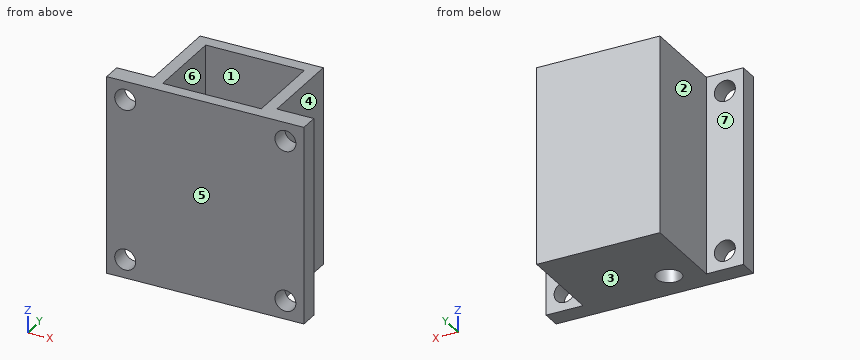
Autodesk Fusion 360 part; units mm, degrees
sketch "Esquisse1" plane through (0, 0, 0) normal (0, 0, 1) x (1, 0, 0)
  line L0 (8, 6.5) -> (-8, 6.5)
  line L1 (-8, 6.5) -> (-8, -6.5)
  line L2 (-8, -6.5) -> (8, -6.5)
  line L3 (8, -6.5) -> (8, 6.5)
  line L4 (8, 6.5) -> (-8, -6.5) construction
  line L5 (-8, 6.5) -> (8, -6.5) construction
  line L6 (-10, -8.5) -> (10, -8.5)
  line L7 (10, -8.5) -> (10, 8.5)
  line L8 (10, 8.5) -> (-10, 8.5)
  line L9 (-10, 8.5) -> (-10, -8.5)
  circle A0 centre (-5, -3.5) radius 2
  dimension "d1" = 16
  dimension "d2" = 13
  dimension "d3" = 2
  dimension "d15" = 4
  dimension "d16" = 3
  dimension "d18" = 3
extrude "Extrusion1" add sketch "Esquisse1" along normal blind 32 contours L6 L7 L8 L9
extrude "Extrusion2" add sketch "Esquisse1" along normal blind 3 contours L0 L1 L2 L3
sketch "Esquisse2" plane through (0, -8.5, 0) normal (0, -1, 0) x (1, 0, 0)
  line L0 (-10, 0) -> (10, 0)
  line L1 (10, 0) -> (10, 32)
  line L2 (10, 32) -> (-10, 32)
  line L3 (-10, 32) -> (-10, 0)
  line L4 (16, 32) -> (-16, 32)
  line L5 (-16, 32) -> (-16, 0)
  line L6 (-16, 0) -> (16, 0)
  line L7 (16, 0) -> (16, 32)
  line L8 (16, 32) -> (-16, 0) construction
  line L9 (-16, 32) -> (16, 0) construction
  line L10 (-10, 0) -> (10, 0)
  circle A0 centre (13, 29) radius 1.7
  line L11 (0, 16) -> (16, 16) construction
  line L12 (0, 16) -> (0, 32) construction
  circle A1 centre (13, 3) radius 1.7
  circle A2 centre (-13, 3) radius 1.7
  circle A3 centre (-13, 29) radius 1.7
  point P0 (0, 16)
  dimension "d8" = 6
  dimension "d9" = 6
  dimension "d10" = 3.4
  dimension "d11" = 3
  dimension "d12" = 3
extrude "Extrusion3" add sketch "Esquisse2" against normal blind 3 contours L3 L4 L5 L6 | L1 L4 L6 L7
equation "d9 = d8"
equation "d18 = d16"
Verification items for the finished model (mm, model axes). Face numbers are marked on the shaded views. A direction names the side the tool comes from. Coordinates: 2 decimals unless noted, no trailing zeros. Order: outer loops, then holes, each group sorted by start corner. A loop starts at its lowest first (then second) coordinate and runs counter-clockwise, first axis right, second up. Notation, with made-up numbers: M -13,48.25 L 21,48.25 A6 ccw 21,53.25 Z; hole C 0,-16 d11. An arc over 180 degrees is marked long. Return JSON: item names as keys, results as strings.
1) Cross-section at A-A, the plane y = -3.5. Record the boundary of the cut face in (x, z).
Answer list:
{"outline": "M -10,0 L -7,0 L -7,3 L -8,3 L -8,32 L -10,32 Z; M -3,0 L 10,0 L 10,32 L 8,32 L 8,3 L -3,3 Z"}
2) Access from +Z, -Z, +X, -X, +Y, -Y to the whole of each face (thin tool, end or side, straight path). Record for the marked faces 5, 6 and 7.
Answer list:
{"face 5": "+Z, -Z, +X, -X, -Y", "face 6": "+Z", "face 7": "+Z, -Z, -X, +Y"}
3) Thickness scan on L1, parallel to Z at x = -13, y = -6.8; L2, parallel to X at y = 0.5, z = 20.5; L3, parallel to Y at x = 2, z = 22.5. Record the ranges inside material, lowest first. Write a range as [from, to].
Answer list:
{"L1": "[0, 1.3], [4.7, 27.3], [30.7, 32]", "L2": "[-10, -8], [8, 10]", "L3": "[-8.5, -6.5], [6.5, 8.5]"}
4) Cross-section at D-D, the plane x = -5. Record the boundary of the cut face in (y, z).
Answer list:
{"outline": "M -8.5,0 L -5.5,0 L -5.5,3 L -6.5,3 L -6.5,32 L -8.5,32 Z; M -1.5,0 L 8.5,0 L 8.5,32 L 6.5,32 L 6.5,3 L -1.5,3 Z"}
5) Gauge pin test, flat ends, axial feed: pin 1 (8 mm diameter, centred on x = -1, y = 0, fed in from -Z); pin 2 (3.5 mm diameter, centred on x = -5, y = -3.5, fed in from +Z); pin 3 (4 mm diameter, centred on x = -2.5, y = 3, fed in from +Z); pin 4 (1.8 mm diameter, centred on x = -13, z = 14, fed in from +Y). Record the tip position at first contact, or that the pin passes through.
Answer list:
{"pin 1": "z = 0", "pin 2": "through", "pin 3": "z = 3", "pin 4": "y = -5.5"}
6) Cross-section at C-C, the plane x = -13. Record the boundary of the cut face in (y, z), and give its area (3 significant figures).
Answer list:
{"outline": "M -8.5,0 L -5.5,0 L -5.5,1.3 L -8.5,1.3 Z; M -8.5,4.7 L -5.5,4.7 L -5.5,27.3 L -8.5,27.3 Z; M -8.5,30.7 L -5.5,30.7 L -5.5,32 L -8.5,32 Z", "area": "75.6 mm2"}
7) Cross-section at B-B, the plane z = 22. Record the boundary of the cut face in (x, y), and give its area (3 significant figures).
Answer list:
{"outline": "M -16,-8.5 L 16,-8.5 L 16,-5.5 L 10,-5.5 L 10,8.5 L -10,8.5 L -10,-5.5 L -16,-5.5 Z; hole M -8,-6.5 L 8,-6.5 L 8,6.5 L -8,6.5 Z", "area": "168 mm2"}
8) Release check for a two-part mould opening along X. For the marked faces 1, 2, 3 and 4 record: +X half, -X half, draft (parallel to the pull), parting line (faces both ways), or undercut.
Answer list:
{"face 1": "undercut", "face 2": "-X half", "face 3": "draft", "face 4": "+X half"}
